The model under review builds one solid part; all positions refer to its coordinate system, in mm. Face numbers are marked on the shaded views. A direction names the side the tool comes from. Give positions to 0.01 mm unless a question says otherwise; leave off trailing zeros. Order: outer loops, then holes, each group sorted by start corner. A loop starts at its lowest first (then second) coordinate and runs counter-clockwise, first axis right, second up. Notation, with made-up numbers: M 30.5,18.25 L 66.5,18.25 A19 cw 66.5,23.25 Z; hole C -9.75,69.5 d1. An arc over 180 degrees is marked long. One line per question, with ' | ' between items. Start each with the question number.
1. For the marked faces 1 and 2, list the 3-axis set-ups (+Z, -Z, +X, -X, +Y, -Y) from which the entire face can be reached by the end or side of a thin tool; tool diameter is ignored.
2. The part is to be moulded in two halves that separate along X. For the marked faces 3, 4 and 5, say which applies: +X half, -X half, draft (parallel to the pull), parting line (faces both ways), or undercut.
3. We need section C-C on x = -15. Write out the cut boundary in (y, z).
4. Wall thickness on L1, parallel to X at y = 4.5, z = 0.5; L2, parallel to Y at x = 2, z = 0.5; L3, parallel to X at y = -2.5, z = 7: over which ranges is each line inside the solid? List them lowest first.
5. We need section D-D on z = 4. Write out the cut boundary in (x, y).
6. We need section B-B on y = 0. Write out the cut boundary in (x, z).
7. We need section A-A on y = 3. Write out the cut boundary in (x, z), then the cut area to 3 significant figures.
8. Insertion check: P1, Ø3, axis at y = 0, z = 5.46, coming from the -X side; P2, Ø8, axis at x = 6, y = 1.5, coming from the +Z side; P3, Ø1.5, axis at x = 1, y = 7.5, coming from the +Z side. Each pin has a flat end and moves straight along its axis. Give the tip position at first contact, or say it passes through.
```python
from build123d import *

# Parameters (mm, degrees)
F0_W      = 28
F0_H      = 18
F1_DEPTH  = 10
F2_T      = 1.5
F3_W      = 7.5
F3_H      = 2.8
F4_DEPTH  = 2
F5_R      = 1.15
F6_DEPTH  = 3
F6_TAPER  = -10
F7_W      = 1.3330084621
F7_H      = 7.0881857659
F7_W_2    = 7
F7_H_2    = 2.3
F8_DEPTH  = 3
F9_R      = 1.8245236246
F10_DEPTH = 5


with BuildPart() as f1:
    # F0 (on Top) → F1 (new body)
    with BuildSketch(Plane.XY):
        with Locations((-2.9748789966, 0.4724050845)):
            Rectangle(F0_W, F0_H)
    extrude(amount=F1_DEPTH)

    # F2
    f2_openings = [f1.faces().sort_by_distance(p)[0] for p in [
        (-2.974879, 0.472405, 10),
    ]]
    offset(amount=F2_T, openings=f2_openings, kind=Kind.INTERSECTION)

    # F3 (on face) → F4 (cut)
    with BuildSketch(Plane.YZ.offset(12.5251210034)):
        with Locations((0, 3.3291981078)):
            Rectangle(F3_W, F3_H)
    extrude(amount=-F4_DEPTH, mode=Mode.SUBTRACT)

    # F5 (on face) → F6 (cut)
    with BuildSketch(Plane(origin=(0, 0, -1.5), x_dir=(1, 0, 0), z_dir=(0, 0, -1))):
        with Locations((-1.3835662976, -6.25)):
            Circle(F5_R)
        with Locations((3.7751210034, -6.1826660439)):
            Circle(F5_R)
    extrude(amount=-F6_DEPTH, taper=F6_TAPER, mode=Mode.SUBTRACT)

    # F7 (on face) → F8 (join)
    with BuildSketch(Plane.XY):
        with Locations((1.1995443201, 5.9283122016)):
            Rectangle(F7_W, F7_H)
        with Locations((-13.4748789966, -7.3775949155)):
            Rectangle(F7_W_2, F7_H_2)
        with Locations((-13.4748789966, 8.3224050845)):
            Rectangle(F7_W_2, F7_H_2)
    extrude(amount=F8_DEPTH)

    # F9 (on face) → F10 (cut)
    with BuildSketch(Plane(origin=(-18.4748789966, 0, 0), x_dir=(0, -1, 0), z_dir=(-1, 0, 0))):
        with Locations((0, 5.4590702057)):
            Circle(F9_R)
    extrude(amount=-F10_DEPTH, mode=Mode.SUBTRACT)


solid = f1.part
```
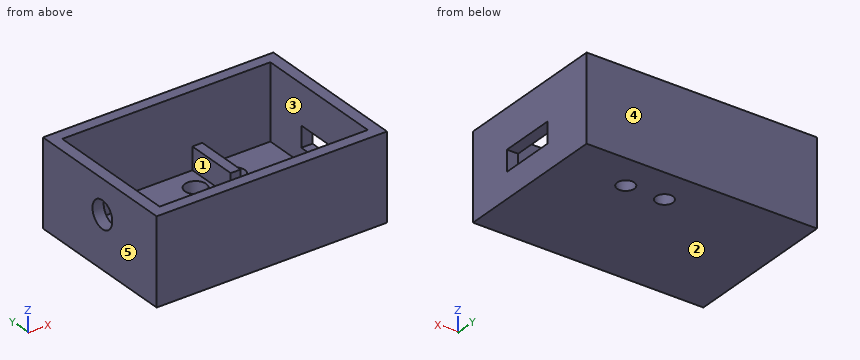
Entries:
1) face 1: +Z | face 2: -Z, +X, -X, +Y, -Y
2) face 3: undercut | face 4: draft | face 5: -X half
3) outline: M -10.03,-1.5 L 10.97,-1.5 L 10.97,10 L 9.47,10 L 9.47,3 L 7.17,3 L 7.17,0 L -6.23,0 L -6.23,3 L -8.53,3 L -8.53,10 L -10.03,10 Z
4) L1: x = -18.47 to -16.97, 0.53 to 1.87, 11.03 to 12.53 | L2: y = -10.03 to -8.53, 9.47 to 10.97 | L3: x = -18.47 to -16.97, 11.03 to 12.53
5) outline: M -18.47,-10.03 L 12.53,-10.03 L 12.53,-3.75 L 11.03,-3.75 L 11.03,-8.53 L -16.97,-8.53 L -16.97,-1.1 L -18.47,-1.1 Z; M -18.47,1.1 L -16.97,1.1 L -16.97,9.47 L 11.03,9.47 L 11.03,3.75 L 12.53,3.75 L 12.53,10.97 L -18.47,10.97 Z
6) outline: M -18.47,-1.5 L 12.53,-1.5 L 12.53,1.93 L 11.03,1.93 L 11.03,0 L -16.97,0 L -16.97,3.63 L -18.47,3.63 Z; M -18.47,7.28 L -16.97,7.28 L -16.97,10 L -18.47,10 Z; M 11.03,4.73 L 12.53,4.73 L 12.53,10 L 11.03,10 Z
7) outline: M -18.47,-1.5 L 12.53,-1.5 L 12.53,1.93 L 11.03,1.93 L 11.03,0 L 1.87,0 L 1.87,3 L 0.53,3 L 0.53,0 L -16.97,0 L -16.97,10 L -18.47,10 Z; M 11.03,4.73 L 12.53,4.73 L 12.53,10 L 11.03,10 Z | area: 76.3 mm^2
8) P1: stops at x = 11.03 | P2: stops at z = 0 | P3: stops at z = 3
